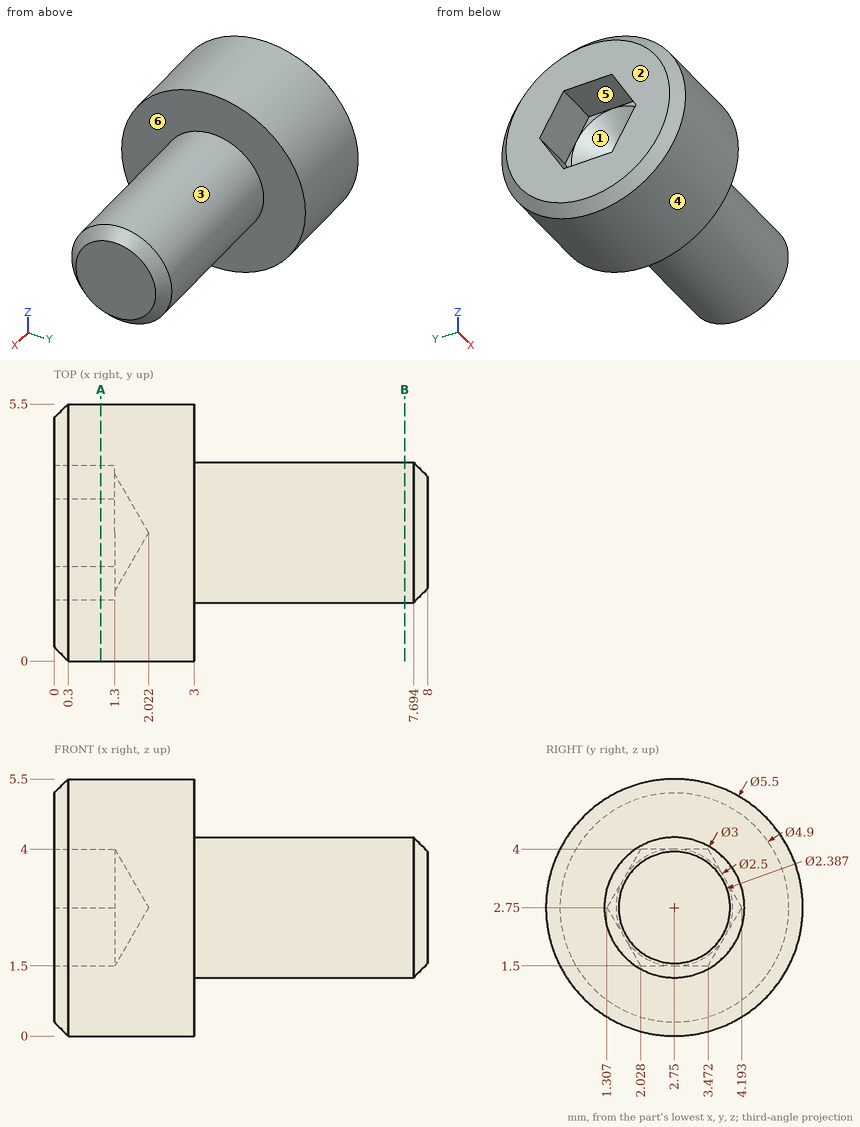
The drawing under review shows one solid part. Ordinate dimensions are in mm from its lowest x, y, z. A direction names the side the tool comes from. Round coordinates to 2 decimals unless told otherwise and drop trailing zeros. Order: outer loops, then holes, each group sorted by start corner. A loop starts at its lowest first (then second) coordinate and runs counter-clockwise, first axis right, second up. Notation, with made-up numbers: (38.25, 86) - (64.25, 86) arc R21 ccw to (64.25, 103) - close; hole circle Ø8 at (-36.5, 51). An arc over 180 degrees is marked (long way). Return JSON: item names as keys, results as strings.
Q1. The part is to be moulded in two halves that separate along Z. For the marked faces 1, 2 and 3, say which applies: pulls with the +Z half, pulls with the -Z half, needs draft (parallel to the pull), parting line crosses it, or undercut.
Computed values:
{"face 1": "undercut", "face 2": "needs draft", "face 3": "parting line crosses it"}
Q2. Consider section B-B on x = 7.5. Write out the cut boundary in (y, z).
Computed values:
{"outline": "circle Ø3 at (2.75, 2.75)"}
Q3. For pin 1 Ø1.5 at (x, y) = (1, 4) entering from +Z; pin 2 Ø0.7 at (y, z) = (3, 2) entering from -X; pin 3 Ø1 at (y, z) = (4.5, 4) entering from +X, all flat-tipped, find the tip position at first contact; note any pin that passes through.
Computed values:
{"pin 1": "stops at z = 5.45", "pin 2": "stops at x = 1.36", "pin 3": "stops at x = 3"}
Q4. Consider section A-A on x = 1. Write out the cut boundary in (y, z).
Computed values:
{"outline": "circle Ø5.5 at (2.75, 2.75); hole (1.31, 2.75) - (2.03, 1.5) - (3.47, 1.5) - (4.19, 2.75) - (3.47, 4) - (2.03, 4) - close"}
Q5. Machinability: for the marked faces 4, 5 and 6, which of the approach directions +Z, -Z, +X, -X, +Y, -Y give a long, thin tool a straight path to every point of the face, cutting with its end or side? Answer none if there is none.
Computed values:
{"face 4": "+X, -X", "face 5": "-X", "face 6": "+X"}
Q6. Wall thickness on L1, parallel to X at y = 1.35, z = 3.6; L2, parallel to X at y = 2.8, z = 2.35; L3, parallel to Z at x = 7, y = 3.8: over which ranges is each line inside the solid? List them lowest first. Write a range as [from, to].
Computed values:
{"L1": "x = [0, 3]", "L2": "x = [1.79, 8]", "L3": "z = [1.68, 3.82]"}
